Autodesk Inventor part; units mm, degrees
ref_plane "YZ Plane" through (0, 0, 0) normal (1, 0, 0) x (0, 1, 0)
ref_plane "XZ Plane" through (0, 0, 0) normal (0, 1, 0) x (-1, 0, 0)
ref_plane "XY Plane" through (0, 0, 0) normal (0, 0, 1) x (1, 0, 0)
sketch "Sketch1" plane through (0, 0, 0) normal (0, 0, 1) x (1, 0, 0)
  circle A0 centre (0, 0) radius 2.75
  circle A1 centre (0, 0) radius 4
  dimension "d0" = 5.5
  dimension "d1" = 8
extrude "Extrusion1" add sketch "Sketch1" along normal blind 20
sketch "Sketch2" plane through (0, 0, 20) normal (0, 0, 1) x (1, 0, 0)
  circle A0 centre (0, 0) radius 7.5
  dimension "d4" = 15
extrude "Extrusion2" add sketch "Sketch2" along normal blind 3
sketch "Sketch3" plane through (0, 0, 0) normal (1, 0, 0) x (0, 1, 0)
  point P0 (0, 0)
sketch "Sketch4" plane through (0, 0, 0) normal (0, 0, -1) x (-1, 0, 0)
  circle A0 centre (0, 0) radius 2.75
  circle A1 centre (0, 0) radius 7.5
  dimension "d7" = 5.5
  dimension "d8" = 15
extrude "Extrusion3" add sketch "Sketch4" along normal blind 3
sketch "Sketch5" plane through (0, 0, -3) normal (0, 0, -1) x (-1, 0, 0)
  circle A0 centre (0, 0) radius 2.75
  circle A1 centre (0, 0) radius 4
extrude "Extrusion4" add sketch "Sketch5" along normal blind 6
sketch "Sketch6" plane through (0, 0, 0) normal (1, 0, 0) x (0, 1, 0)
  circle A0 centre (0, -6) radius 1.5
  line L0 (-4, -9) -> (4, -9)
  point P0 (0, 0)
  dimension "d13" = 3
  dimension "d14" = 3
extrude "Extrusion5" add sketch "Sketch6" along normal blind 6
sketch "Sketch7" plane through (6, 0, -6) normal (1, 0, 0) x (0, 0, -1)
  circle A0 centre (0, 0) radius 1.5
  circle A1 centre (0, 0) radius 1.5
  point P0 (-6, 0)
  dimension "d17" = 3
extrude "Extrusion6" cut sketch "Sketch7" against normal blind 20
sketch "Sketch8" plane through (0, 0, -3) normal (0, 0, -1) x (-1, 0, 0)
  line L0 (-5, 3) -> (-2.75, 3)
  line L1 (-2.75, 3) -> (-2.75, -3)
  line L2 (-2.75, -3) -> (-5, -3)
  line L3 (-5, -3) -> (-5, 3)
  line L4 (2.75, -3) -> (5, -3)
  line L5 (5, -3) -> (5, 3)
  line L6 (5, 3) -> (2.75, 3)
  line L7 (2.75, 3) -> (2.75, -3)
  point P0 (0, 0)
  dimension "d20" = 3
  dimension "d21" = 3
  dimension "d22" = 5
  dimension "d23" = 2.75
  dimension "d24" = 2.75
  dimension "d25" = 5
extrude "Extrusion7" add sketch "Sketch8" along normal blind 6
sketch "Sketch9" plane through (5, -3, -3) normal (1, 0, 0) x (0, 0, -1)
  arc A0 (1.5, 3) -> (4.5, 3) centre (3, 3) ccw
  point P0 (-3, 3)
hole "Hole1" at (5, 0, -6) direction (-1, 0, 0) diameter 3 depth 8 tip angle 118
sketch "Sketch10" plane through (-5, -3, -3) normal (-1, 0, 0) x (0, 0, 1)
  circle A0 centre (-3, 3) radius 1.5
  point P0 (3, 3)
hole "Hole2" at (-5, 0, -6) direction (1, 0, 0) diameter 3 depth 8 tip angle 118
thread "Thread1"
properties part number "bearing v1"
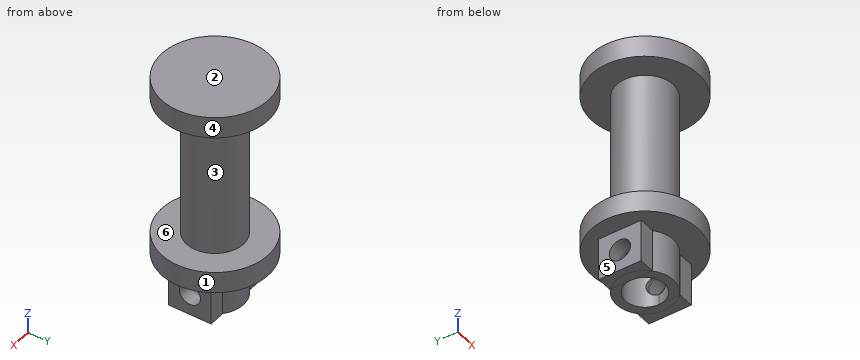
Can you work these out from the model? Positions are in its coordinate system, mm. Face numbers are marked on the shaded views. A direction names the side the tool comes from. Coordinates: 2 decimals unless noted, no trailing zeros. Loops run counter-clockwise (first coordinate to the right, second up) from the corner with the lowest first, then second, coordinate; pieces in that order, holes last.
Item 1: Suppose I cut it at D-D (z = 16). Please give me the cut outline in (x, y), then the cut area to 3 significant figures.
Answers below:
outline: circle Ø8 at (0, 0); hole circle Ø5.5 at (0, 0)
area: 26.5 mm2
Item 2: Which directions (+Z, -Z, +X, -X, +Y, -Y) give clear straight access to the entire face, cutting with the end or side of a thin tool? Please do the marked faces 4, 5 and 6.
Answers below:
face 4: +Z, -Z
face 5: -Z, -X, +Y, -Y
face 6: none
Item 3: Please list where these lines run through material, in increasing order: L1, parallel to Y at x = -4.5, z = -6; L2, parallel to Z at x = 1, y = -5.75; L3, parallel to Y at x = 0, z = 7.
Answers below:
L1: y = -3 to -1.5, 1.5 to 3
L2: z = -3 to 0, 20 to 23
L3: y = -4 to -2.75, 2.75 to 4
Item 4: Suppose I cut it at B-B (y = 5.5). Please give me the cut outline in (x, z).
Answers below:
outline: (-5.1, -3) - (5.1, -3) - (5.1, 0) - (-5.1, 0) - close; (-5.1, 20) - (5.1, 20) - (5.1, 23) - (-5.1, 23) - close
Item 5: Suppose I cut it at A-A (z = -6). Please give me the cut outline in (x, y), then the cut area to 3 significant figures.
Answers below:
outline: (-5, -3) - (-2.75, -3) - (-2.75, -2.9) arc R4 ccw to (2.75, -2.9) - (2.75, -3) - (5, -3) - (5, -1.5) - (2.3, -1.5) arc R2.75 cw to (-2.3, -1.5) - (-5, -1.5) - close; (-5, 1.5) - (-2.3, 1.5) arc R2.75 cw to (2.3, 1.5) - (5, 1.5) - (5, 3) - (2.75, 3) - (2.75, 2.9) arc R4 ccw to (-2.75, 2.9) - (-2.75, 3) - (-5, 3) - close
area: 29.1 mm2
Item 6: I'm going to push flat-ended pins straight in: pin 1 (4.5 mm diameter, centred on x = -1, y = 0, fed in from -Z); pin 2 (1.5 mm diameter, centred on x = 2, z = 5, fed in from +Y); pin 3 (5 mm diameter, centred on y = 0, z = -6, fed in from +X); pin 4 (1 mm diameter, centred on x = -5, z = -1, fed in from -Y). Where does each tip first touch, or does it pass through?
Answers below:
pin 1: stops at z = -9
pin 2: stops at y = 3.8
pin 3: stops at x = 5
pin 4: stops at y = -6
Item 7: If we mould it in two halves opening along Z, with no side actions, what happens to the marked faces 1, 2 and 3? For each: released by +Z, released by -Z, zero draft, split by the parting line, or undercut.
Answers below:
face 1: zero draft
face 2: released by +Z
face 3: undercut
Item 8: Suppose I cut it at C-C (x = 6.25). Please give me the cut outline in (y, z), then the cut area to 3 significant figures.
Answers below:
outline: (-4.15, -3) - (4.15, -3) - (4.15, 0) - (-4.15, 0) - close; (-4.15, 20) - (4.15, 20) - (4.15, 23) - (-4.15, 23) - close
area: 49.7 mm2
